Build history of the part. All positions in model axes, mm. A direction names the side the tool comes from. Give positions to 0.01 mm unless a question says otherwise; leave off trailing zeros. Order: outer loops, then holes, each group sorted by start corner. A loop starts at its lowest first (then second) coordinate and runs counter-clockwise, first axis right, second up. Notation, with made-up numbers: (-27, 68.5) -> (9, 68.5) arc R33 ccw to (9, 100.5) -> close; hole circle Ø11 at (5, 6). An arc over 180 degrees is marked (long way). Write item = value, one per line. Start each with the question number.
from build123d import *

# Parameters (mm, degrees)
F0_W     = 127
F0_H     = 50.8
F1_DEPTH = 38.1
F2_R     = 25.39999
F3_R     = 12.2082879552
F3_R_2   = 12.7
F4_DEPTH = 19.05


# Not quite as in the source:
# - a fillet or chamfer is up to 0.001 mm smaller than in the source, because OpenCascade refuses the exact size


with BuildPart() as f1:
    # F0 (on Front) → F1 (new body)
    with BuildSketch(Plane.XZ):
        Rectangle(F0_W, F0_H)
    extrude(amount=F1_DEPTH)

    # F2 (radius 25.4 in the source; OpenCascade refuses exactly that, so slightly less here)
    f2_edges = [f1.edges().sort_by_distance(p)[0] for p in [
        (63.5, -19.05, 25.4),
        (63.5, -19.05, -25.4),
        (-63.5, -19.05, 25.4),
        (-63.5, -19.05, -25.4),
    ]]
    fillet(f2_edges, radius=F2_R)

    # F3 (on face) → F4 (cut)
    with BuildSketch(Plane(origin=(0, 0, 0), x_dir=(-1, 0, 0), z_dir=(0, 1, 0))):
        with Locations((47.625, 0)):
            Circle(F3_R)
        with Locations((-47.625, 0)):
            Circle(F3_R_2)
    extrude(amount=-F4_DEPTH, mode=Mode.SUBTRACT)


solid = f1.part
(1) Flat gauge pins, fed straight in: P1, Ø10, axis at y = -21.5, z = -18.5, coming from the +X side; P2, Ø1.5, axis at y = -12.5, z = -2.5, coming from the +X side; P3, Ø1.5, axis at y = -33.5, z = 15.5, coming from the -X side. Where does each tip first touch, or does it go through?
(2) Cut at D-D, the plane x = -53. Give the cut face in (y, z).
(3) Cut at A-A, the plane y = -5. Give the number of separate pieces and of enclosed holes in the cut face, plus the area to 3 significant figures.
(4) Mould opens along X. For faces 3 (the face through (-1, -38.1, 0)), 4 (the face through (55.86, -19.32, -18.16)), 5 (the face through (-35.43, -9.39, 0.54)) say: released by +X, released by -X, zero draft, split by the parting line, or undercut.
(5) Cut at C-C, the plane z = 8.5. Give the cut face in (x, y).
(6) 3-axis set-ups, long thin cutter, end or side, ignore diameter. For faces 1 (the face through (48, -19.05, 0)), 2 (the face through (-1, -19, 25.4)): which of +Z, -Z, +X, -X, +Y, -Y reach the whole face in a straight line?
(7) Wall check: line 1 (X direction, y = -5.5, z = 3); line 2 (X direction, y = -7.5, z = -2.5); line 3 (Y direction, x = -48.5, z = -6). Give the ranges that are in metal, low to high. Write a range as [from, to].
Results:
q1.P1 = 59.62
q1.P2 = 63.44
q1.P3 = -58.78
q2.outline = (-38.1, -20.57) -> (0, -20.57) -> (0, -10.96) -> (-19.05, -10.96) -> (-19.05, 10.96) -> (0, 10.96) -> (0, 20.57) -> (-38.1, 20.57) -> close
q3.separate_pieces = 1
q3.enclosed_holes = 2
q3.area = 4,920 mm2
q4.face_3 = zero draft
q4.face_4 = released by +X
q4.face_5 = undercut
q5.outline = (-62.04, -38.1) -> (62.04, -38.1) -> (62.04, 0) -> (57.06, 0) -> (57.06, -19.05) -> (38.19, -19.05) -> (38.19, 0) -> (-38.86, 0) -> (-38.86, -19.05) -> (-56.39, -19.05) -> (-56.39, 0) -> (-62.04, 0) -> close
q6.face_1 = +Y
q6.face_2 = +Z, +X, -X, +Y, -Y
q7.line_1 = [-63.32, -59.46], [-35.79, 35.28], [59.97, 63.32]
q7.line_2 = [-63.38, -59.57], [-35.68, 35.17], [60.08, 63.38]
q7.line_3 = [-38.1, -19.05]
